from build123d import *

# Parameters (mm, degrees)
SKETCH1_W           = 81.28
SKETCH1_H           = 68.58
BOSS_EXTRUDE1_DEPTH = 1.6
CHAMFER1_SIZE       = 2.54
CUT_EXTRUDE1_REACH  = 55.197
SKETCH2_R           = 0.65
SKETCH2_R_2         = 1.4
SKETCH2_R_3         = 1.175
LPATTERN1_COUNT     = 4
LPATTERN1_PITCH     = 20


with BuildPart() as part:
    # Sketch1 → Boss-Extrude1 (new body)
    with BuildSketch(Plane(origin=(0, 0, 0), x_dir=(1, 0, 0), z_dir=(0, 1, 0))):
        Rectangle(SKETCH1_W, SKETCH1_H)
    extrude(amount=BOSS_EXTRUDE1_DEPTH)

    # Chamfer1
    chamfer1_edges = [part.edges().sort_by_distance(p)[0] for p in [
        (-40.64, 0.8, -34.29),
        (40.64, 0.8, -34.29),
    ]]
    chamfer(chamfer1_edges, length=CHAMFER1_SIZE)

    # Sketch2 → Cut-Extrude1 (cut, up to next)
    with BuildSketch(Plane.XZ, mode=Mode.PRIVATE) as cut_extrude1_sk1:
        with Locations(Location((-29.87, 29.29, 0), (0, 0, 270))):
            Circle(SKETCH2_R)
    cut_extrude1_tool1 = extrude(cut_extrude1_sk1.sketch, amount=-CUT_EXTRUDE1_REACH, mode=Mode.PRIVATE) & part.part
    # Sketch2 → Cut-Extrude1 (cut, up to next)
    with BuildSketch(Plane.XZ, mode=Mode.PRIVATE) as cut_extrude1_sk2:
        with Locations(Location((-37.37, 29.29, 0), (0, 0, 270))):
            Circle(SKETCH2_R_2)
    cut_extrude1_tool2 = extrude(cut_extrude1_sk2.sketch, amount=-CUT_EXTRUDE1_REACH, mode=Mode.PRIVATE) & part.part
    # Sketch2 → Cut-Extrude1 (cut, up to next)
    with BuildSketch(Plane.XZ, mode=Mode.PRIVATE) as cut_extrude1_sk3:
        with Locations(Location((-22.37, 29.29, 0), (0, 0, 270))):
            Circle(SKETCH2_R_2)
    cut_extrude1_tool3 = extrude(cut_extrude1_sk3.sketch, amount=-CUT_EXTRUDE1_REACH, mode=Mode.PRIVATE) & part.part
    # Sketch2 → Cut-Extrude1 (cut, up to next)
    with BuildSketch(Plane.XZ, mode=Mode.PRIVATE) as cut_extrude1_sk4:
        with Locations(Location((-37.37, 25.29, 0), (0, 0, 270))):
            Circle(SKETCH2_R_3)
    cut_extrude1_tool4 = extrude(cut_extrude1_sk4.sketch, amount=-CUT_EXTRUDE1_REACH, mode=Mode.PRIVATE) & part.part
    # Sketch2 → Cut-Extrude1 (cut, up to next)
    with BuildSketch(Plane.XZ, mode=Mode.PRIVATE) as cut_extrude1_sk5:
        with Locations(Location((-22.37, 25.29, 0), (0, 0, 270))):
            Circle(SKETCH2_R_3)
    cut_extrude1_tool5 = extrude(cut_extrude1_sk5.sketch, amount=-CUT_EXTRUDE1_REACH, mode=Mode.PRIVATE) & part.part
    cut_extrude1_1 = cut_extrude1_tool1.solids().sort_by_distance((-29.87, 0, 29.29))[0]
    add(cut_extrude1_1, mode=Mode.SUBTRACT)
    cut_extrude1_2 = cut_extrude1_tool2.solids().sort_by_distance((-37.37, 0, 29.29))[0]
    add(cut_extrude1_2, mode=Mode.SUBTRACT)
    cut_extrude1_3 = cut_extrude1_tool3.solids().sort_by_distance((-22.37, 0, 29.29))[0]
    add(cut_extrude1_3, mode=Mode.SUBTRACT)
    cut_extrude1_4 = cut_extrude1_tool4.solids().sort_by_distance((-37.37, 0, 25.29))[0]
    add(cut_extrude1_4, mode=Mode.SUBTRACT)
    cut_extrude1_5 = cut_extrude1_tool5.solids().sort_by_distance((-22.37, 0, 25.29))[0]
    add(cut_extrude1_5, mode=Mode.SUBTRACT)
    cut_extrude1 = cut_extrude1_1 + cut_extrude1_2 + cut_extrude1_3 + cut_extrude1_4 + cut_extrude1_5  # Cut-Extrude1 as one shape, for the pattern or mirror that repeats it

    # LPattern1: Cut-Extrude1 ×4
    with Locations(*[(i * LPATTERN1_PITCH, 0, 0) for i in range(1, LPATTERN1_COUNT)]):
        add(cut_extrude1, mode=Mode.SUBTRACT)


solid = part.part
Can you work these out from the model? Positions are in its coordinate system, mm. Give positions to 0.01 mm unless a question says otherwise; leave off trailing zeros. Loops run counter-clockwise (first coordinate to the right, second up) from the corner with the lowest first, then second, coordinate; pieces in that order, holes last. Notation, with made-up numbers: (35, -14) -> (48, -14) arc R32 cw to (48, 18) -> close; hole circle Ø4 at (-28, 52). An arc over 180 degrees is marked (long way). Use one line per item in the form item = value.
1) If we section it at A-A (x = -17.37): Please give me the cut outline in (y, z) (3 decimals), plus the area to 3 significant figures.
Answers:
outline = (0, -34.29) -> (1.6, -34.29) -> (1.6, 24.115) -> (0, 24.115) -> close; (0, 26.465) -> (1.6, 26.465) -> (1.6, 27.89) -> (0, 27.89) -> close; (0, 30.69) -> (1.6, 30.69) -> (1.6, 34.29) -> (0, 34.29) -> close
area = 101 mm²
2) We'd pull the mould along Z, two halves only. Please class faces 1 (the face through (-1, 1, 34.29)), 2 (the face through (-1, 1.6, 0)), 3 (the face through (18.6, 0.8, 30.3)): released by +Z, released by -Z, zero draft, split by the parting line, or undercut.
Answers:
face_1 = released by +Z
face_2 = zero draft
face_3 = undercut
3) If we section it at B-B (y = 0.9): Count the separate pieces of the cut face and the enclosed holes in it, plus the area to 3 significant figures.
Answers:
separate_pieces = 1
enclosed_holes = 20
area = 5,480 mm²
4) I need wall thicknesses on line 1 along Z through (x, y) = (37.5, 1.15); line 2 along Z through (x, y) = (-29.5, 0.3). Which ranges of each line are inside material? Lowest first, please.
Answers:
line_1 = -34.29 to 24.12, 26.46 to 27.9, 30.68 to 34.29
line_2 = -34.29 to 28.76, 29.82 to 34.29
